Here's the drawing with two shaded views (mm, measured from the low corner). I have some questions. Coordinates: 2 decimals unless noted, no trailing zeros. Order: outer loops, then holes, each group sorted by start corner. A loop starts at its lowest first (then second) coordinate and runs counter-clockwise, first axis right, second up. Notation, with made-up numbers: (-6, 56.5) -> (-2, 56.5) arc R11 ccw to (-2, 72.5) -> close; hole circle Ø1 at (53.5, -0.5). An arc over 180 degrees is marked (long way). Return JSON: item names as keys, results as strings. Group by question number.
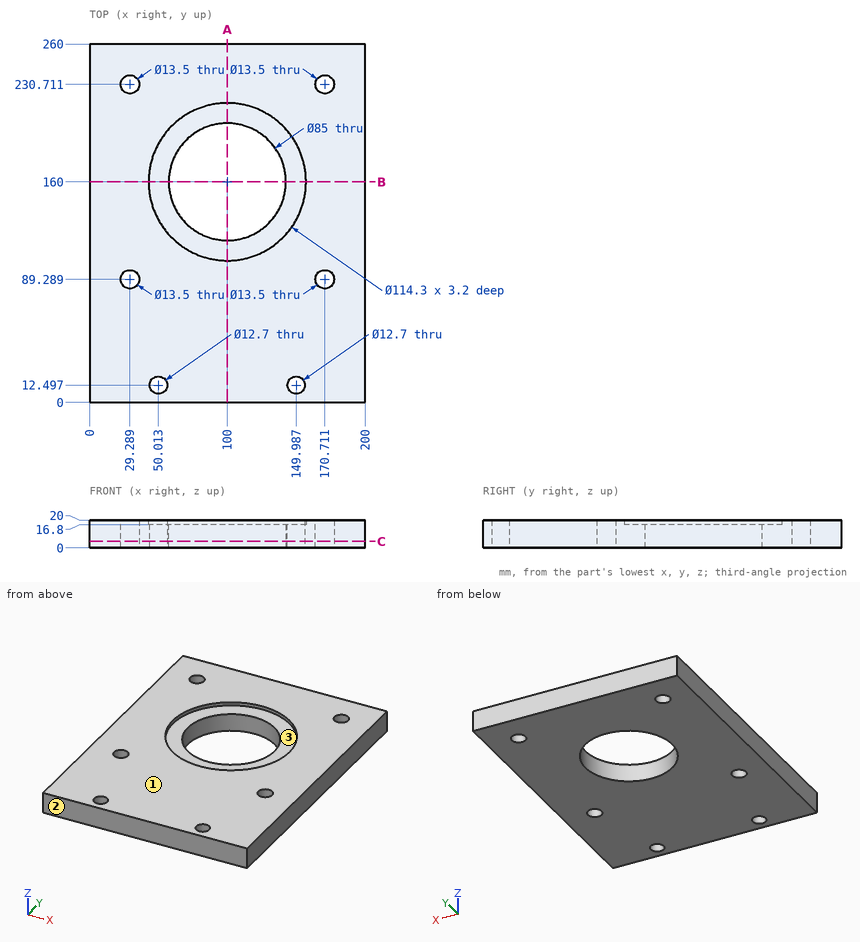
Q1. I'm going to push a flat-ended pin straight in: pin 1 Ø10 at (x, y) = (149.99, 12.5) entering from -Z. Where does the tip first touch, or does it pass through?
Q2. I need wall thicknesses on line 1 along Y through (x, z) = (170, 6.5); line 2 along Y through (x, z) = (100, 19); line 3 along X through (y, z) = (85, 6) (1 decimal). Which ranges of each line are inside material? Lowest first, please. Write a range as from..to.
Q3. I want a section at A-A on x = 100. Please give me the cut outline in (y, z).
Q4. I want a section at C-C on z = 4.75. Please give me the cut outline in (x, y).
Q5. I want a section at B-B on y = 160. Please give me the cut outline in (x, z).
Q6. We'd pull the mould along Y, two halves only. Please class the marked faces 1, 2 and 3: pulls with the +Y half, pulls with the -Y half, needs draft (parallel to the pull), parting line crosses it, or undercut.
Response values:
{
 "1": {"pin 1": "passes through"},
 "2": {"line 1": "y = 0..82.58, 96..224, 237.42..260", "line 2": "y = 0..102.85, 217.15..260", "line 3": "x = 0..24.1, 34.5..165.5, 175.9..200"},
 "3": {"outline": "(0, 0) -> (117.5, 0) -> (117.5, 16.8) -> (102.85, 16.8) -> (102.85, 20) -> (0, 20) -> close; (202.5, 0) -> (260, 0) -> (260, 20) -> (217.15, 20) -> (217.15, 16.8) -> (202.5, 16.8) -> close"},
 "4": {"outline": "(0, 0) -> (200, 0) -> (200, 260) -> (0, 260) -> close; hole circle Ø13.5 at (29.29, 89.29); hole circle Ø13.5 at (29.29, 230.71); hole circle Ø12.7 at (50.01, 12.5); hole circle Ø85 at (100, 160); hole circle Ø12.7 at (149.99, 12.5); hole circle Ø13.5 at (170.71, 89.29); hole circle Ø13.5 at (170.71, 230.71)"},
 "5": {"outline": "(0, 0) -> (57.5, 0) -> (57.5, 16.8) -> (42.85, 16.8) -> (42.85, 20) -> (0, 20) -> close; (142.5, 0) -> (200, 0) -> (200, 20) -> (157.15, 20) -> (157.15, 16.8) -> (142.5, 16.8) -> close"},
 "6": {"face 1": "needs draft", "face 2": "pulls with the -Y half", "face 3": "undercut"}
}
